Read the model definition and answer for the solid it produces. Units are mm, in the model's axes. Round coordinates to 2 decimals unless told otherwise and drop trailing zeros. Order: outer loops, then holes, each group sorted by start corner. A loop starts at its lowest first (then second) coordinate and runs counter-clockwise, first axis right, second up. Notation, with made-up numbers: (87.25, 83.25) - (92.25, 83.25) arc R26 ccw to (92.25, 115.25) - close; hole circle Ø7 at (43.5, 38). An arc over 180 degrees is marked (long way). Answer as a JSON object with one key per item and string values. Group by question number.
Q1. Given pin 1 Ø2 at (x, z) = (580.5, 3) entering from -Y; pin 2 Ø0.6 at (y, z) = (4, -0.5) entering from +X, each flat-ended and moving along its own axis, determine where each tip first touches the part or whether it passes through.
Q2. Consider line 1 (X direction, y = 4.5, z = -2); line 2 (X direction, y = -1.25, z = 4.5); line 3 (Y direction, x = 98, z = -0.25). Determine where each line is inside the solid, lowest interval first.
Q3. A cutting plane is placed at B-B on x = 619. Determine the outline of the cut face in (y, z), and give its area (3 significant figures).
Q4. A cutting plane is placed at A-A on x = 63.5. Determine the outline of the cut face in (y, z), and give its area (3 significant figures).
```python
from build123d import *

# Parameters (mm, degrees)
SKICA2_R                 = 5
ODEBRAT_VYSUNUT_M1_DEPTH = 5
SKICA3_W                 = 15
SKICA3_H                 = 10
ODEBRAT_VYSUNUT_M2_DEPTH = 16


with BuildPart() as part:
    # Skica1 → Rotovat3 (revolve)
    with BuildSketch(Plane.XY, mode=Mode.PRIVATE) as rotovat3_sk:
        Polygon((301.25, 5), (0, 5), (0, 0), (745.975022487, 0), (745.975001326, 2.5), (301.25, 2.5), align=None)
    revolve(rotovat3_sk.sketch.rotate(Axis((256.066983307, 0, 0), (1, 0, 0)), 90), axis=Axis((256.066983307, 0, 0), (1, 0, 0)))

    # Skica2 → Odebrat vysunutím1 (cut)
    with BuildSketch(Plane.ZY):
        Circle(SKICA2_R)
    extrude(amount=-ODEBRAT_VYSUNUT_M1_DEPTH, mode=Mode.SUBTRACT)

    # Skica3 → Odebrat vysunutím2 (cut)
    with BuildSketch(Plane(origin=(0, 19, 0), x_dir=(1, 0, 0), z_dir=(0, 1, 0))):
        with Locations((20.207259422, 0)):
            Rectangle(SKICA3_W, SKICA3_H)
    extrude(amount=-ODEBRAT_VYSUNUT_M2_DEPTH, mode=Mode.SUBTRACT)


solid = part.part
```
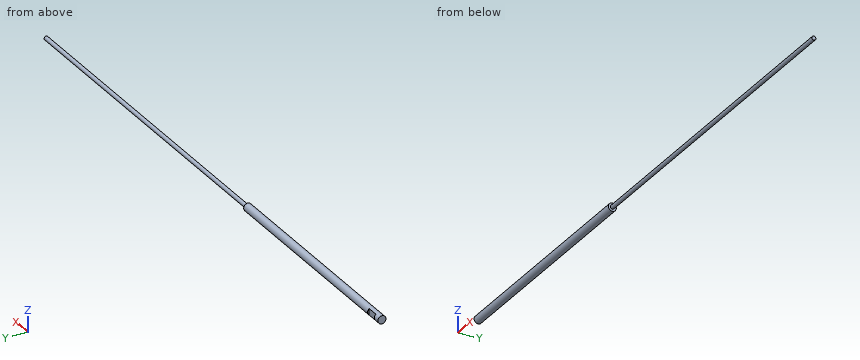
Result set:
{
 "1": {"pin 1": "stops at y = -1.5", "pin 2": "stops at x = 301.25"},
 "2": {"line 1": "x = 5 to 12.71, 27.71 to 301.25", "line 2": "x = 5 to 301.25", "line 3": "y = -4.99 to 4.99"},
 "3": {"outline": "circle Ø5 at (0, 0)", "area": "19.6 mm²"},
 "4": {"outline": "circle Ø10 at (0, 0)", "area": "78.5 mm²"}
}
